Verification items for the finished model (mm, model axes). A direction names the side the tool comes from. Give positions to 0.01 mm unless a question says otherwise; leave off trailing zeros. Write each loop counter-clockwise with the first axis right and the second up, starting at its lowest first coordinate (ties: lowest second). Pieces come first, ordered by that corner, then holes. Notation, with made-up numbers: (71, 35.5) -> (93, 35.5) arc R17 cw to (93, 47.5) -> close; hole circle Ø5 at (16, 57). An arc over 180 degrees is marked (long way). Use CSV: the item, a comma, the result in double quotes. Start each with the question number.
```python
from build123d import *

# Parameters (mm, degrees)
SKETCH1_W           = 54
SKETCH1_H           = 26
SKETCH1_W_2         = 29.9
SKETCH1_H_2         = 8.9
BOSS_EXTRUDE1_DEPTH = 4.6
SKETCH2_W           = 3.6
SKETCH2_H           = 8.9
BOSS_EXTRUDE2_DEPTH = 1.8
SKETCH3_R           = 3.45
BOSS_EXTRUDE3_DEPTH = 7.4
SKETCH4_W           = 54
SKETCH4_H           = 26
SKETCH4_W_2         = 48
SKETCH4_H_2         = 20
BOSS_EXTRUDE4_DEPTH = 8.9
SKETCH5_W           = 51
SKETCH5_H           = 23
SKETCH5_W_2         = 48
SKETCH5_H_2         = 20
CUT_EXTRUDE1_DEPTH  = 3
SKETCH6_R           = 1.6
CUT_EXTRUDE2_DEPTH  = 12
CUT_EXTRUDE3_REACH  = 40.525
SKETCH7_W           = 12.16
SKETCH7_H           = 10.9
SKETCH8_R           = 3
CUT_EXTRUDE4_DEPTH  = 34.401384702
CHAMFER1_SIZE       = 1.5


with BuildPart() as part:
    # Sketch1 → Boss-Extrude1 (new body)
    with BuildSketch(Plane.XY):
        with Locations((0, -2.95)):
            Rectangle(SKETCH1_W, SKETCH1_H)
        with Locations((0, -5.5)):
            Rectangle(SKETCH1_W_2, SKETCH1_H_2, mode=Mode.SUBTRACT)
    extrude(amount=BOSS_EXTRUDE1_DEPTH)

    # Sketch2 → Boss-Extrude2 (add)
    with BuildSketch(Plane.XY.offset(4.6)):
        with Locations((4.25, -5.5)):
            Rectangle(SKETCH2_W, SKETCH2_H)
    extrude(amount=-BOSS_EXTRUDE2_DEPTH)

    # Sketch3 → Boss-Extrude3 (add)
    with BuildSketch(Plane(origin=(0, 0, 0), x_dir=(-1, 0, 0), z_dir=(0, 0, -1))):
        with Locations(Location((-18.5, -5.5, 0), (0, 0, 270))):
            Circle(SKETCH3_R)
        with Locations(Location((18.5, -5.5, 0), (0, 0, 270))):
            Circle(SKETCH3_R)
    extrude(amount=BOSS_EXTRUDE3_DEPTH)

    # Sketch4 → Boss-Extrude4 (add)
    with BuildSketch(Plane(origin=(0, 0, 0), x_dir=(-1, 0, 0), z_dir=(0, 0, -1))):
        with Locations((0, -2.95)):
            Rectangle(SKETCH4_W, SKETCH4_H)
        with Locations((0, -2.95)):
            Rectangle(SKETCH4_W_2, SKETCH4_H_2, mode=Mode.SUBTRACT)
    extrude(amount=BOSS_EXTRUDE4_DEPTH)

    # Sketch5 → Cut-Extrude1 (cut)
    with BuildSketch(Plane(origin=(0, 0, -8.9), x_dir=(-1, 0, 0), z_dir=(0, 0, -1))):
        with Locations((0, -2.95)):
            Rectangle(SKETCH5_W, SKETCH5_H)
        with Locations((0, -2.95)):
            Rectangle(SKETCH5_W_2, SKETCH5_H_2, mode=Mode.SUBTRACT)
    extrude(amount=-CUT_EXTRUDE1_DEPTH, mode=Mode.SUBTRACT)

    # Sketch6 → Cut-Extrude2 (cut)
    with BuildSketch(Plane(origin=(0, 0, -7.4), x_dir=(-1, 0, 0), z_dir=(0, 0, -1))):
        with Locations(Location((-18.5, -5.5, 0), (0, 0, 90))):
            Circle(SKETCH6_R)
        with Locations(Location((18.5, -5.5, 0), (0, 0, 90))):
            Circle(SKETCH6_R)
    extrude(amount=-CUT_EXTRUDE2_DEPTH, mode=Mode.SUBTRACT)

    # Cut-Extrude3: up to this face of the body (flat: up to its plane)
    cut_extrude3_end = Plane(part.part.faces().sort_by_distance((0, 7.05, -2.95))[0])
    # Sketch7 → Cut-Extrude3 (cut, up to the picked face)
    with BuildSketch(Plane(origin=(0, 10.05, 0), x_dir=(1, 0, 0), z_dir=(0, 1, 0)), mode=Mode.PRIVATE) as cut_extrude3_sk1:
        with Locations((0, 3.45)):
            Rectangle(SKETCH7_W, SKETCH7_H)
    cut_extrude3_tool1 = split(extrude(cut_extrude3_sk1.sketch, amount=-CUT_EXTRUDE3_REACH, mode=Mode.PRIVATE), bisect_by=cut_extrude3_end, keep=Keep.BOTH, mode=Mode.PRIVATE)
    add(cut_extrude3_tool1.solids().sort_by(Axis((0, 10.05, -3.45), (0, -1, 0)))[0], mode=Mode.SUBTRACT)

    # Sketch8 → Cut-Extrude4 (cut, through all)
    with BuildSketch(Plane.XY.offset(2.6)):
        with Locations((-18.5, -5.5)):
            Circle(SKETCH8_R)
        with Locations((18.5, -5.5)):
            Circle(SKETCH8_R)
    extrude(amount=CUT_EXTRUDE4_DEPTH, mode=Mode.SUBTRACT)

    # Chamfer1
    # the kernel refuses this chamfer: 1.5 mm, written as the material it takes off along each edge
    with BuildSketch(Plane(origin=(-18.5, -5.5, 2.6), x_dir=(0, 1, 0), z_dir=(-1, 0, 0))) as chamfer1_piece_1_section:
        Polygon((1.6 + CHAMFER1_SIZE, 0), (1.6, CHAMFER1_SIZE), (1.6, 0), align=None)
    chamfer1_piece_1 = revolve(axis=Axis((-18.5, -5.5, 2.6), (0, 0, -1)), mode=Mode.PRIVATE)
    chamfer1_piece_1 = chamfer1_piece_1 & Plane(origin=(-18.5, -5.5, 1.79661682), x_dir=(1, 0, 0), z_dir=(0, 0, -1)) * Cylinder(3, 13, mode=Mode.PRIVATE)
    add(chamfer1_piece_1, mode=Mode.SUBTRACT)
    with BuildSketch(Plane(origin=(18.5, -5.5, 2.6), x_dir=(0, 1, 0), z_dir=(-1, 0, 0))) as chamfer1_piece_2_section:
        Polygon((1.6 + CHAMFER1_SIZE, 0), (1.6, CHAMFER1_SIZE), (1.6, 0), align=None)
    chamfer1_piece_2 = revolve(axis=Axis((18.5, -5.5, 2.6), (0, 0, -1)), mode=Mode.PRIVATE)
    chamfer1_piece_2 = chamfer1_piece_2 & Plane(origin=(18.5, -5.5, 1.79661682), x_dir=(1, 0, 0), z_dir=(0, 0, -1)) * Cylinder(3, 13, mode=Mode.PRIVATE)
    add(chamfer1_piece_2, mode=Mode.SUBTRACT)


solid = part.part
```
(1) Thickness scan on line 1 (X direction, y = -5.5, z = -3.75); line 2 (X direction, y = 4.25, z = -6.75); line 3 (Y direction, x = 5, z = 1.25). Record the ranges inside material, lowest first. Write a range as from..to.
(2) Section check D-D on x = 4. Record the cut outline in (y, z).
(3) Draft check along Y on faces 1 (the face through (-15, 7.05, -3)), 2 (the face through (0.4, 10.05, 2.4)), 3 (the face through (6.08, 9, -3)). Enter one of: released by +Y, released by -Y, zero draft, split by the parting line, or undercut.
(4) Go/stop test with flat-tipped pins: pin 1 (1 mm diameter, centred on x = 1.5, y = -6.5, fed in from +Z) (1 decimal); pin 2 (1.1 mm diameter, centred on x = 4.5, y = -5.5, fed in from -Z); pin 3 (11.5 mm diameter, centred on x = 1.5, y = 0, fed in from -Z); pin 4 (6.5 mm diameter, centred on x = -4, z = -3, fed in from +Y). Record where each tip stops, or that it passes through.
(5) Section check A-A on z = -4.5. Record the cut outline in (x, y).
(6) Set-up check for faces 4 (the face through (14.95, -6, 2)), 5 (the face through (0, 7.05, 1)), 6 (the face through (15.08, -5.05, -3.65)): record each of +Z, -Z, +X, -X, +Y, -Y from which the full face is reachable in a straight line by a thin tool's end or side.
(7) Section check C-C on y = 0.25. Record the cut outline in (x, z), then the cut area to 3 significant figures.
(8) Section check B-B on x = -8. Record the cut outline in (y, z).
Data:
1,line 1,"x = -27..-24, -21.95..-20.1, -16.9..-15.05, 15.05..16.9, 20.1..21.95, 24..27"
1,line 2,"x = -27..-25.5, 25.5..27"
1,line 3,"y = -15.95..-9.95, -1.05..7.05"
2,outline,"(-15.95, -8.9) -> (-14.45, -8.9) -> (-14.45, -5.9) -> (-12.95, -5.9) -> (-12.95, 0) -> (-9.95, 0) -> (-9.95, 2.8) -> (-1.05, 2.8) -> (-1.05, 0) -> (7.05, 0) -> (7.05, 2) -> (10.05, 2) -> (10.05, 4.6) -> (-15.95, 4.6) -> close"
3,face 1,"undercut"
3,face 2,"released by +Y"
3,face 3,"zero draft"
4,pin 1,"passes through"
4,pin 2,"stops at z = 2.8"
4,pin 3,"stops at z = 0"
4,pin 4,"stops at y = 10.05"
5,outline,"(-27, -15.95) -> (27, -15.95) -> (27, 10.05) -> (6.08, 10.05) -> (6.08, 7.05) -> (24, 7.05) -> (24, -12.95) -> (-24, -12.95) -> (-24, 7.05) -> (-6.08, 7.05) -> (-6.08, 10.05) -> (-27, 10.05) -> close; circle Ø6.9 at (-18.5, -5.5); circle Ø6.9 at (18.5, -5.5); hole circle Ø3.2 at (-18.5, -5.5); hole circle Ø3.2 at (18.5, -5.5)"
6,face 4,"+Z, -Z"
6,face 5,"-Z, +Y"
6,face 6,"-Z"
7,outline,"(-27, -8.9) -> (-25.5, -8.9) -> (-25.5, -5.9) -> (-24, -5.9) -> (-24, 0) -> (24, 0) -> (24, -5.9) -> (25.5, -5.9) -> (25.5, -8.9) -> (27, -8.9) -> (27, 4.6) -> (-27, 4.6) -> close"
7,area,"293 mm2"
8,outline,"(-15.95, -8.9) -> (-14.45, -8.9) -> (-14.45, -5.9) -> (-12.95, -5.9) -> (-12.95, 0) -> (-9.95, 0) -> (-9.95, 4.6) -> (-15.95, 4.6) -> close; (-1.05, 0) -> (7.05, 0) -> (7.05, -5.9) -> (8.55, -5.9) -> (8.55, -8.9) -> (10.05, -8.9) -> (10.05, 4.6) -> (-1.05, 4.6) -> close"
